from build123d import *

# Parameters (mm, degrees)
F1_DEPTH = 304.8
F2_R     = 5.08
F4_DEPTH = 25.4
F5_R     = 9.525
F6_DEPTH = 25.4


with BuildPart() as f1:
    # F0 (on Front) → F1 (new body, symmetric)
    with BuildSketch(Plane.XZ):
        Polygon((0, 76.2), (0, 0), (76.2, 0), (76.2, 6.35), (6.35, 6.35), (6.35, 76.2), align=None)
    extrude(amount=F1_DEPTH, both=True)

    # F2
    f2_edges = [f1.edges().sort_by_distance(p)[0] for p in [
        (6.35, 0, 76.2),
        (6.35, 0, 6.35),
        (76.2, 0, 6.35),
    ]]
    fillet(f2_edges, radius=F2_R)

    # F3 (on face) → F4 (cut)
    with BuildSketch(Plane(origin=(0, 0, 0), x_dir=(0, -1, 0), z_dir=(-1, 0, 0))):
        Polygon((-304.8, 116.164517), (-304.8, 6.35), (-194.985483, 116.164517), align=None)
    extrude(amount=-F4_DEPTH, mode=Mode.SUBTRACT)

    # F5 (on face) → F6 (cut)
    with BuildSketch(Plane(origin=(0, 0, 0), x_dir=(1, 0, 0), z_dir=(0, 0, -1))):
        with Locations((38.1, 254)):
            Circle(F5_R)
        with Locations((38.1, 146.05)):
            Circle(F5_R)
    extrude(amount=-F6_DEPTH, mode=Mode.SUBTRACT)


solid = f1.part
Geometry check sheet. Reference: the model listing, model coordinates, mm. A direction names the side the tool comes from. Round coordinates to 2 decimals unless told otherwise and drop trailing zeros. Write each loop counter-clockwise with the first axis right and the second up, starting at its lowest first coordinate (ties: lowest second). Pieces come first, ordered by that corner, then holes. Notation, with made-up numbers: (-29.75, 4) -> (24.25, 4) arc R22 ccw to (24.25, 27) -> close; hole circle Ø1 at (-12, -5). An arc over 180 degrees is marked (long way). One line per item, written item: value. Start each with the question number.
(1) Draft check along X on faces 3 (the cylindrical face through (36.04, -136.75, 3.13)), 4 (the flat face through (0, -4, 39)), 5 (the flat face through (38, -4, 0)). Enter one of: +X half, -X half, draft (parallel to the pull), parting line (faces both ways), or undercut.
(2) Cross-section at C-C, the plane y = 249. Record the cut outline in (x, z), and give its area (3 significant figures).
(3) Cross-section at D-D, the plane x = 64.5. Record the cut outline in (y, z).
(4) Access from +Z, -Z, +X, -X, +Y, -Y to the whole of each face (thin tool, end or side, straight path). Record for faces 1 (the flat face through (42, -4, 6.35)), 2 (the flat face through (3.09, 270.36, 40.79)).
(5) Cross-section at B-B, the plane y = -146.05. Record the cut outline in (x, z) (3 decimals).
(6) Scan lines: line 1 (Y direction, x = 38.1, z = 5) (3 decimals); line 2 (X direction, y = -254, z = 2.25) (3 decimals); line 3 (Z direction, x = 25, y = -59). Record each from-to range of solid material in increasing order. Write a range as [from, to].
(7) Go/stop test with flat-tipped pins: pin 1 Ø25 at (x, y) = (38.1, -254) entering from +Z; pin 2 Ø8 at (x, y) = (52.5, 69) entering from +Z; pin 3 Ø4 at (y, z) = (-51, 52.5) entering from +X. Record where each tip stops, or that it passes through.
(8) Cross-section at A-A, the plane x = 38.1. Record the cut outline in (y, z) (3 decimals).
Answer:
1. face 3: undercut
1. face 4: -X half
1. face 5: draft
2. outline: (0, 0) -> (76.2, 0) -> (76.2, 1.27) arc R5.08 ccw to (71.12, 6.35) -> (11.43, 6.35) arc R5.08 cw to (6.35, 11.43) -> (6.35, 62.15) -> (0, 62.15) -> close
2. area: 838 mm²
3. outline: (-304.8, 0) -> (304.8, 0) -> (304.8, 6.35) -> (-304.8, 6.35) -> close
4. face 1: +Z, +X, +Y, -Y
4. face 2: +Z, +X, -X, +Y
5. outline: (0, 0) -> (28.575, 0) -> (28.575, 6.35) -> (11.43, 6.35) arc R5.08 cw to (6.35, 11.43) -> (6.35, 71.12) arc R5.08 ccw to (1.27, 76.2) -> (0, 76.2) -> close; (47.625, 0) -> (76.2, 0) -> (76.2, 1.27) arc R5.08 ccw to (71.12, 6.35) -> (47.625, 6.35) -> close
6. line 1: [-304.8, -263.525], [-244.475, -155.575], [-136.525, 304.8]
6. line 2: [0, 28.575], [47.625, 76.105]
6. line 3: [0, 6.35]
7. pin 1: z = 6.35
7. pin 2: z = 6.35
7. pin 3: x = 6.35
8. outline: (-304.8, 0) -> (-263.525, 0) -> (-263.525, 6.35) -> (-304.8, 6.35) -> close; (-244.475, 0) -> (-155.575, 0) -> (-155.575, 6.35) -> (-244.475, 6.35) -> close; (-136.525, 0) -> (304.8, 0) -> (304.8, 6.35) -> (-136.525, 6.35) -> close
